```python
from build123d import *

# Parameters (mm, degrees)
F1_DEPTH       = 15.875
F3_D           = 7.62
F3_CSINK_D     = 15.24
F3_CSINK_ANGLE = 90
F4_R           = 6.35
F5_SIZE        = 0.635


with BuildPart() as f1:
    # F0 (on Top) → F1 (new body)
    with BuildSketch(Plane.XY):
        Polygon((130.175, 0), (0, 0), (0, -15.875), (130.175, -60.325), align=None)
    extrude(amount=F1_DEPTH)

    # F3 (through all)
    with Locations(Plane.XY.offset(15.875)):
        with Locations((35.439426, -11.131202), (94.735574, -22.225)):
            CounterSinkHole(F3_D / 2, F3_CSINK_D / 2, counter_sink_angle=F3_CSINK_ANGLE)

    # F4
    f4_edges = [f1.edges().sort_by_distance(p)[0] for p in [
        (0, -15.875, 7.9375),
        (0, 0, 7.9375),
        (130.175, -60.325, 7.9375),
        (130.175, 0, 7.9375),
    ]]
    fillet(f4_edges, radius=F4_R)

    # F5
    f5_edges = [f1.edges().sort_by_distance(p)[0] for p in [
        (65.0875, 0, 0),
        (128.315128, -1.859872, 0),
        (1.859872, -1.859872, 0),
        (130.175, -28.898358, 0),
        (0, -8.84165, 0),
        (127.519085, -56.611619, 0),
        (1.185096, -15.027386, 0),
        (63.035537, -37.39933, 0),
        (90.925574, -22.225, 0),
        (31.629426, -11.131202, 0),
    ]]
    chamfer(f5_edges, length=F5_SIZE)


solid = f1.part
```
Here's how the part is built. I have some questions about the finished solid (model axes, mm). Give positions to 0.01 mm unless a question says otherwise; leave off trailing zeros. Loops run counter-clockwise (first coordinate to the right, second up) from the corner with the lowest first, then second, coordinate; pieces in that order, holes last. Notation, with made-up numbers: M 24.25,-38.75 L 64.25,-38.75 A15 ccw 64.25,-21.75 Z; hole C 5,-4 d9. An arc over 180 degrees is marked long. Put each result on its own line as item: value. Start each with the question number.
(1) I want a section at A-A on z = 5.75. Please give me the cut outline in (x, y) (3 decimals).
(2) If we mould it in two halves opening along X, with no side actions, what happens to faces 1 (the flat face through (62.32, -36.81, 0.31)), 2 (the conical face through (90.925, -21.025, 12.25)), 3 (the flat face through (66, 0, 8))? For each: +X half, -X half, draft (parallel to the pull), parting line (faces both ways), or undercut.
(3) Will these pins go through, and if not, where does the flat tip stop? pin 1 Ø2 at (x, y) = (55.5, -37.5) entering from -Z; pin 2 Ø6 at (x, z) = (70, 13.5) entering from -Y.
(4) I need wall thicknesses on line 1 along X through (y, z) = (-11, 11.75) (3 decimals); line 2 along Y through (x, z) = (72, 1); line 3 along Y through (x, z) = (108, 15). Which ranges of each line are inside material? Lowest first, please. Write a range as [from, to].
(5) I want a section at C-C on y = -37. Please give me the cut outline in (x, z) (3 decimals).
(6) I want a section at B-B on x = 71. Please give me the cut outline in (y, z) (3 decimals).
Answer block:
1. outline: M 0,-11.333 A6.35 ccw 4.298,-17.343 L 121.773,-57.456 A6.35 ccw 130.175,-51.447 L 130.175,-6.35 A6.35 ccw 123.825,0 L 6.35,0 A6.35 ccw 0,-6.35 Z; hole C 35.439,-11.131 d7.62; hole C 94.736,-22.225 d7.62
2. face 1: -X half
2. face 2: undercut
2. face 3: draft
3. pin 1: through
3. pin 2: y = -40.8
4. line 1: [0, 31.632], [39.247, 130.175]
4. line 2: [-40.46, 0]
4. line 3: [-52.75, 0]
5. outline: M 61.866,0.635 L 63.831,0 L 129.54,0 L 130.175,0.635 L 130.175,15.875 L 61.866,15.875 Z
6. outline: M -40.119,0.635 L -39.448,0 L -0.635,0 L 0,0.635 L 0,15.875 L -40.119,15.875 Z
